Part print with two shaded views. Sizes in mm from the minimum x, y, z corner. A direction names the side the tool comes from. Round coordinates to 2 decimals unless told otherwise and drop trailing zeros. Order: outer loops, then holes, each group sorted by start corner. A loop starts at its lowest first (then second) coordinate and runs counter-clockwise, first axis right, second up. Notation, with made-up numbers: M 87.25,12.5 L 95.25,12.5 A21 ccw 95.25,19.5 Z; hole C 73,-18.75 d3. An arc over 180 degrees is marked long. Return JSON: item names as keys, results as strings. Group by question number.
Item 1: Slice it at C-C on y = 5.5. Write the cut outline in (x, z), then the cut area to 3 significant figures.
Item 2: Slice it at A-A on z = 7. Write the cut outline in (x, y).
Item 3: Probe line 1 along Z through (x, y) = (12.5, 0.3); line 2 along X through (y, z) = (37, 38). List the from-to ranges inside material, lowest first.
Item 4: Slice it at B-B on x = 12.5. Write the cut outline in (y, z).
Item 5: Slice it at D-D on y = 29. Write the cut outline in (x, z), then the cut area to 3 significant figures.
Item 6: Which spindle directions (+Z, -Z, +X, -X, +Y, -Y) get a long thin tool onto all of the face, cutting with end or side? Do the marked faces 1 and 2. Say none if no direction does.
Item 7: Pin check, flat tips, straight feed: pin 1 Ø1.5 at (x, z) = (7.5, 14) entering from +Y; pin 2 Ø7 at (y, z) = (5.5, 21) entering from +X. Stop position of each tip, or through.
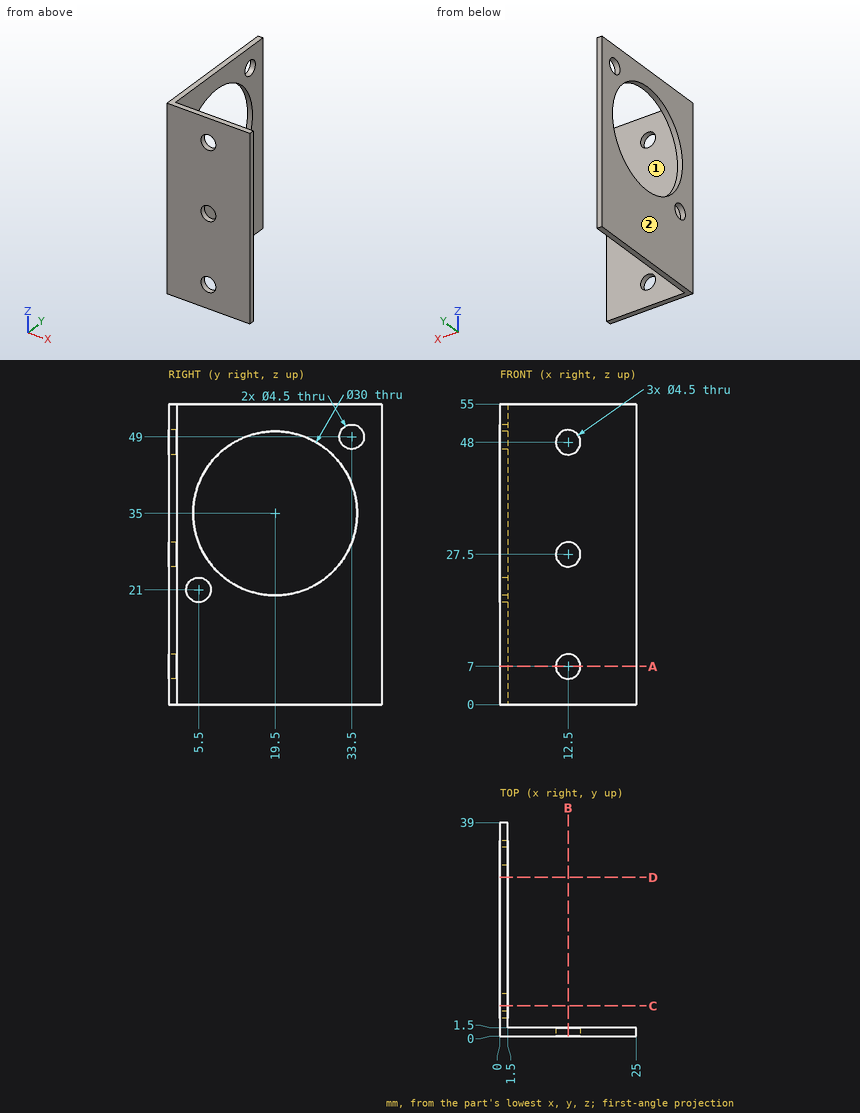
Output values:
{
 "1": {"outline": "M 0,0 L 1.5,0 L 1.5,18.75 L 0,18.75 Z; M 0,23.25 L 1.5,23.25 L 1.5,29.61 L 0,29.61 Z; M 0,40.39 L 1.5,40.39 L 1.5,55 L 0,55 Z", "area": "59.6 mm²"},
 "2": {"outline": "M 0,0 L 10.25,0 L 10.25,1.5 L 1.5,1.5 L 1.5,39 L 0,39 Z; M 14.75,0 L 25,0 L 25,1.5 L 14.75,1.5 Z"},
 "3": {"line 1": "0 to 4.75, 9.25 to 25.25, 29.75 to 45.75, 50.25 to 55", "line 2": "0 to 1.5"},
 "4": {"outline": "M 0,0 L 1.5,0 L 1.5,4.75 L 0,4.75 Z; M 0,9.25 L 1.5,9.25 L 1.5,25.25 L 0,25.25 Z; M 0,29.75 L 1.5,29.75 L 1.5,45.75 L 0,45.75 Z; M 0,50.25 L 1.5,50.25 L 1.5,55 L 0,55 Z"},
 "5": {"outline": "M 0,0 L 1.5,0 L 1.5,23.39 L 0,23.39 Z; M 0,46.61 L 1.5,46.61 L 1.5,55 L 0,55 Z", "area": "47.7 mm²"},
 "6": {"face 1": "+Z, -Z, +X, +Y", "face 2": "+Z, -Z, -X, +Y, -Y"},
 "7": {"pin 1": "y = 1.5", "pin 2": "x = 1.5"}
}
